from build123d import *

# Parameters (mm, degrees)
BOSS_EXTRUDE1_DEPTH  = 10
M4_CLEARANCE_HOLE1_D = 4.5
M2_CLEARANCE_HOLE1_D = 2.4


with BuildPart() as part:
    # Sketch1 → Boss-Extrude1 (new body, symmetric)
    with BuildSketch(Plane.XY):
        Polygon((0, 0), (0, 12.7), (1.6002, 12.7), (1.6002, 1.6002), (12.7, 1.6002), (12.7, 0), align=None)
    extrude(amount=BOSS_EXTRUDE1_DEPTH, both=True)

    # M4 Clearance Hole1 (through all)
    with Locations(Plane(origin=(0, 1.6002, 0), x_dir=(1, 0, 0), z_dir=(0, 1, 0))):
        with Locations((7.7, -5), (7.7, 5)):
            Hole(M4_CLEARANCE_HOLE1_D / 2)

    # M2 Clearance Hole1 (through all)
    with Locations(Plane.ZY):
        with Locations((-6.35, 8.7), (6.35, 8.7)):
            Hole(M2_CLEARANCE_HOLE1_D / 2)


solid = part.part
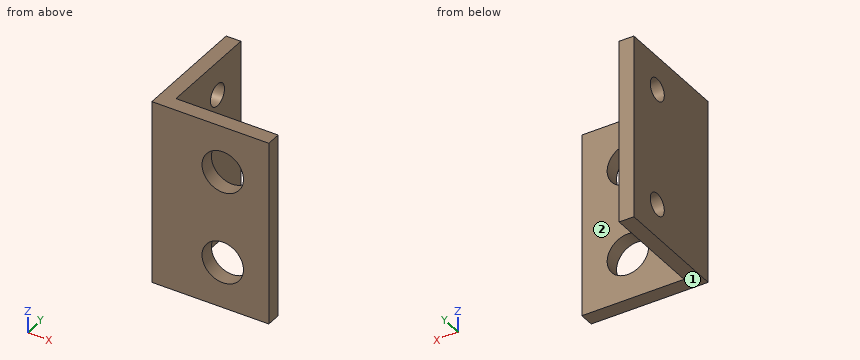
Model file for the job. Use its own axes, mm. Face numbers are marked on the shaded views. A direction names the side the tool comes from. Give positions to 0.01 mm unless a question says otherwise; leave off trailing zeros. Order: outer loops, then holes, each group sorted by start corner. A loop starts at its lowest first (then second) coordinate and runs counter-clockwise, first axis right, second up. Notation, with made-up numbers: (-15.75, 27.25) - (17.25, 27.25) arc R25 ccw to (17.25, 57.25) - close; hole circle Ø7 at (-9, 76). An arc over 180 degrees is marked (long way). Return JSON: item names as keys, results as strings.
1) Flat gauge pins, fed straight in: P1, Ø4, axis at x = 5, z = 3, coming from the -Y side; P2, Ø1, axis at x = 8, z = -4.5, coming from the +Y side; P3, Ø7, axis at x = 7.7, z = -5, coming from the +Y side. Where does each tip first touch, or does it go through?
Geometry says:
{"P1": "y = 0", "P2": "through", "P3": "y = 1.6"}
2) Cut at C-C, the plane x = 7.7. Give the cut face in (y, z), plus the area to 3 significant figures.
Geometry says:
{"outline": "(0, -10) - (1.6, -10) - (1.6, -7.25) - (0, -7.25) - close; (0, -2.75) - (1.6, -2.75) - (1.6, 2.75) - (0, 2.75) - close; (0, 7.25) - (1.6, 7.25) - (1.6, 10) - (0, 10) - close", "area": "17.6 mm²"}
3) 3-axis set-ups, long thin cutter, end or side, ignore diameter. For the marked faces 1 and 2: which of +Z, -Z, +X, -X, +Y, -Y reach the whole face in a straight line?
Geometry says:
{"face 1": "-Z, +X, -X, +Y, -Y", "face 2": "+Z, -Z, +X, +Y"}
4) Cut at B-B, the plane z = -6.35. Give the cut face in (x, y), plus the area to 3 significant figures.
Geometry says:
{"outline": "(0, 0) - (5.9, 0) - (5.9, 1.6) - (1.6, 1.6) - (1.6, 7.5) - (0, 7.5) - close; (0, 9.9) - (1.6, 9.9) - (1.6, 12.7) - (0, 12.7) - close; (9.5, 0) - (12.7, 0) - (12.7, 1.6) - (9.5, 1.6) - close", "area": "28.5 mm²"}
5) Probe line 1 (Z direction, x = 7.7, y = 0.5); line 2 (Y direction, x = 0.8, z = -6.35); line 3 (X direction, y = 7.25, z = -3). List the from-to ranges inside material, lowest first. Write a range as from..to.
Geometry says:
{"line 1": "-10..-7.25, -2.75..2.75, 7.25..10", "line 2": "0..7.5, 9.9..12.7", "line 3": "0..1.6"}
6) Cut at D-D, the plane z = 4.5. Give the cut face in (x, y), plus the area to 3 significant figures.
Geometry says:
{"outline": "(0, 0) - (5.51, 0) - (5.51, 1.6) - (1.6, 1.6) - (1.6, 12.7) - (0, 12.7) - close; (9.89, 0) - (12.7, 0) - (12.7, 1.6) - (9.89, 1.6) - close", "area": "31.1 mm²"}
7) Cut at A-A, the plane y = 8.7. Give the cut face in (x, z), plus the area to 3 significant figures.
Geometry says:
{"outline": "(0, -10) - (1.6, -10) - (1.6, -7.55) - (0, -7.55) - close; (0, -5.15) - (1.6, -5.15) - (1.6, 5.15) - (0, 5.15) - close; (0, 7.55) - (1.6, 7.55) - (1.6, 10) - (0, 10) - close", "area": "24.3 mm²"}
